Geometry: final body of the model. Coordinates: model frame, mm. Face numbers are marked on the shaded views. Give positions to 0.01 mm unless a question says otherwise; leave off trailing zeros. Write each loop counter-clockwise with the first axis right and the second up, starting at its lowest first coordinate (ties: lowest second). Pieces come first, ordered by that corner, then holes.
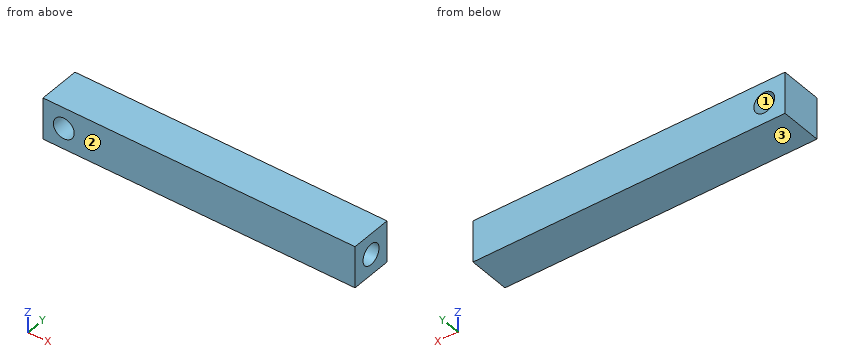
```python
from build123d import *

# Parameters (mm, degrees)
SKETCH1_W               = 40
SKETCH1_H               = 40
BOSS_EXTRUDE1_DEPTH     = 300
CUT_EXTRUDE1_DEPTH      = 100
CUT_EXTRUDE1_DEPTH_BACK = 100
SKETCH2_R               = 10
CUT_EXTRUDE2_DEPTH      = 50
CUT_EXTRUDE2_DEPTH_BACK = 50
SKETCH3_R               = 10
SKETCH4_W               = 40
SKETCH4_H               = 40
BOSS_EXTRUDE2_DEPTH     = 300
CUT_EXTRUDE3_DEPTH      = 80
CUT_EXTRUDE3_DEPTH_BACK = 80
SKETCH5_R               = 10
SKETCH6_R               = 10
CUT_EXTRUDE4_DEPTH      = 30


with BuildPart() as part:
    # Sketch1 → Boss-Extrude1 (new body)
    with BuildSketch(Plane(origin=(0, 0, 0), x_dir=(0, 0, -1), z_dir=(1, 0, 0))):
        Rectangle(SKETCH1_W, SKETCH1_H)
    extrude(amount=BOSS_EXTRUDE1_DEPTH)

    # Sketch2 → Cut-Extrude1 (cut, two sides: drawn at the far end of the back side and taken through both)
    with BuildSketch(Plane(origin=(0, 0, 0), x_dir=(1, 0, 0), z_dir=(0, 1, 0)).offset(-CUT_EXTRUDE1_DEPTH_BACK)):
        with Locations(Location((20, 0, 0), (0, 0, 270))):
            Circle(SKETCH2_R)
    extrude(amount=CUT_EXTRUDE1_DEPTH + CUT_EXTRUDE1_DEPTH_BACK, mode=Mode.SUBTRACT)

    # Sketch3 → Cut-Extrude2 (cut, two sides: drawn at the far end of the back side and taken through both)
    with BuildSketch(Plane(origin=(300, 0, 0), x_dir=(0, 0, -1), z_dir=(1, 0, 0)).offset(-CUT_EXTRUDE2_DEPTH_BACK)):
        Circle(SKETCH3_R)
    extrude(amount=CUT_EXTRUDE2_DEPTH + CUT_EXTRUDE2_DEPTH_BACK, mode=Mode.SUBTRACT)

    # Sketch4 → Boss-Extrude2 (add)
    with BuildSketch(Plane(origin=(0, 0, 0), x_dir=(0, 0, -1), z_dir=(1, 0, 0))):
        Rectangle(SKETCH4_W, SKETCH4_H)
    extrude(amount=BOSS_EXTRUDE2_DEPTH)

    # Sketch5 → Cut-Extrude3 (cut, two sides: drawn at the far end of the back side and taken through both)
    with BuildSketch(Plane(origin=(0, 0, 0), x_dir=(1, 0, 0), z_dir=(0, 1, 0)).offset(-CUT_EXTRUDE3_DEPTH_BACK)):
        with Locations(Location((20, 0, 0), (0, 0, 270))):
            Circle(SKETCH5_R)
    extrude(amount=CUT_EXTRUDE3_DEPTH + CUT_EXTRUDE3_DEPTH_BACK, mode=Mode.SUBTRACT)

    # Sketch6 → Cut-Extrude4 (cut)
    with BuildSketch(Plane(origin=(300, 0, 0), x_dir=(0, 0, -1), z_dir=(1, 0, 0))):
        Circle(SKETCH6_R)
    extrude(amount=-CUT_EXTRUDE4_DEPTH, mode=Mode.SUBTRACT)


solid = part.part
```
Item 1: Section B-B, the plane y = 0. Return the cut outline in (x, z).
Found:
outline: (0, -20) - (300, -20) - (300, -10) - (270, -10) - (270, 10) - (300, 10) - (300, 20) - (0, 20) - close; hole circle Ø20 at (20, 0)
Item 2: Section A-A, the plane x = 20. Return the cut outline in (y, z), plus the area to 3 significant figures.
Found:
outline: (-20, -20) - (20, -20) - (20, -10) - (-20, -10) - close; (-20, 10) - (20, 10) - (20, 20) - (-20, 20) - close
area: 800 mm2
Item 3: Pin query (flat end, axial travel): pin 1 Ø16 at (y, z) = (0, 0) entering from +X. Return the tip coordinate at first contact, or that it passes through.
Found:
pin 1: stops at x = 270
Item 4: Pull-direction query (Z, two-part tool) for the marked faces 1, 2 and 3; classes: +Z half, -Z half, draft (parallel to the pull), parting line (faces both ways), or undercut.
Found:
face 1: undercut
face 2: draft
face 3: -Z half
Item 5: Section D-D, the plane y = -13. Return the cut outline in (x, z).
Found:
outline: (0, -20) - (300, -20) - (300, 20) - (0, 20) - close; hole circle Ø20 at (20, 0)
Item 6: Line query: L1, parallel to Y at x = 284.75, z = 0; L2, parallel to X at y = 8, z = 0. Output: solid intervals per line, ascending.
Found:
L1: y = -20 to -10, 10 to 20
L2: x = 0 to 10, 30 to 270
Item 7: Section C-C, the plane z = 0. Return the cut outline in (x, y), plus the area to 3 significant figures.
Found:
outline: (0, -20) - (10, -20) - (10, 20) - (0, 20) - close; (30, -20) - (300, -20) - (300, -10) - (270, -10) - (270, 10) - (300, 10) - (300, 20) - (30, 20) - close
area: 10,600 mm2
